Could you check a few things on this model? Use its own coordinates, in mm. Give positions to 0.01 mm unless a question says otherwise; leave off trailing zeros. Loops run counter-clockwise (first coordinate to the right, second up) from the corner with the lowest first, then second, coordinate; pieces in that order, holes last. Notation, with made-up numbers: (10.25, 30) - (52.25, 30) arc R11 ccw to (52.25, 34) - close; hole circle Ø7 at (-12, -1.5). An arc over 180 degrees is marked (long way). Write each question's results on one line, items separated by ' | '. Start each with the question number.
(1) Suppose I cut it at C-C (x = -19.5). Count the separate pieces of the cut face and the enclosed holes in it, and give its area (3 significant figures).
(2) Suppose I cut it at D-D (y = 1.5). Please give me the cut outline in (x, z) (1 decimal), and give its area (3 significant figures).
(3) Suppose I cut it at A-A (z = 8.5). Please give me the cut outline in (x, y), and give its area (3 significant figures).
(4) Suppose I cut it at B-B (y = 5.25). Please give me the cut outline in (x, z) (1 decimal).
(5) I need wall thicknesses on line 1 (Z direction, x = -19.5, y = 5); line 2 (X direction, y = 3.5, z = -13.5) (3 decimals); line 3 (X direction, y = 1.5, z = -14). Which ranges of each line are inside material? Lowest first, please.
(6) If we mould it in two halves opening along X, with no side actions, what happens to faces 1 (the face through (-6.331, 3.131, -14.795)), 2 (the face through (-13.7, 4.8, -13.9)), 3 (the face through (-16, 6.35, 0))? For each: released by +X, released by -X, zero draft, split by the parting line, or undercut.
(7) For pin 1 (7 mm diameter, centred on x = -20.18, z = -13.16, fed in from +Y); pin 2 (12.5 mm diameter, centred on x = -15.8, z = 5.57, fed in from -Y); pin 3 (12 mm diameter, centred on x = -13, z = -12, fed in from -Y), each with a flat end and sliding along its axis, tell me the tip position at first contact or that it passes through.
from build123d import *

# Parameters (mm, degrees)
BOSS_EXTRUDE1_DEPTH                               = 6.35
CSK_FOR_8_FLAT_HEAD_MACHINE_SCREW_100_D           = 4.4958
CSK_FOR_8_FLAT_HEAD_MACHINE_SCREW_100_CSINK_D     = 8.4328
CSK_FOR_8_FLAT_HEAD_MACHINE_SCREW_100_CSINK_ANGLE = 100
SKETCH2_R                                         = 82.042
CUT_EXTRUDE1_DEPTH                                = 43.217023873
SKETCH5_R                                         = 1.1303
CUT_EXTRUDE2_DEPTH                                = 35.271884391
SKETCH6_R                                         = 4.7625
CUT_EXTRUDE3_DEPTH                                = 35.271884391


with BuildPart() as part:
    # Sketch1 → Boss-Extrude1 (new body)
    with BuildSketch(Plane(origin=(0, 0, 0), x_dir=(1, 0, 0), z_dir=(0, 1, 0))):
        Polygon((-28.511825699, 11.575271113), (-22.161825699, 17.925271113), (-9.461825699, 17.925271113), (-3.111825699, 11.575271113), (-3.111825699, -12.554728887), (-28.511825699, -12.554728887), align=None)
    extrude(amount=BOSS_EXTRUDE1_DEPTH)

    # CSK for #8 Flat Head Machine Screw (100)1 (through all)
    with Locations(Plane(origin=(0, 6.35, 0), x_dir=(1, 0, 0), z_dir=(0, 1, 0))):
        with Locations((-20.177450699, 13.162771113), (-11.446200699, 13.162771113)):
            CounterSinkHole(CSK_FOR_8_FLAT_HEAD_MACHINE_SCREW_100_D / 2, CSK_FOR_8_FLAT_HEAD_MACHINE_SCREW_100_CSINK_D / 2, counter_sink_angle=CSK_FOR_8_FLAT_HEAD_MACHINE_SCREW_100_CSINK_ANGLE)

    # Sketch2 → Cut-Extrude1 (cut, through all)
    with BuildSketch(Plane.XY.offset(12.554728887)):
        with Locations((-15.811825699, -81.053067579)):
            Circle(SKETCH2_R)
    extrude(amount=-CUT_EXTRUDE1_DEPTH, mode=Mode.SUBTRACT)

    # Sketch5 → Cut-Extrude2 (cut, through all)
    with BuildSketch(Plane(origin=(0, 6.35, 0), x_dir=(1, 0, 0), z_dir=(0, 1, 0))):
        with Locations(Location((-15.799380503, -5.569728887, 0), (0, 0, 270))):
            Circle(SKETCH5_R)
    extrude(amount=-CUT_EXTRUDE2_DEPTH, mode=Mode.SUBTRACT)

    # Sketch6 → Cut-Extrude3 (cut, through all)
    with BuildSketch(Plane(origin=(0, 6.35, 0), x_dir=(1, 0, 0), z_dir=(0, 1, 0))):
        with Locations(Location((-15.799380503, -5.569728887, 0), (0, 0, 270))):
            Circle(SKETCH6_R)
    extrude(amount=-CUT_EXTRUDE3_DEPTH, mode=Mode.SUBTRACT)


solid = part.part
Output values:
1) separate pieces: 3 | enclosed holes: 0 | area: 107 mm2
2) outline: (-28.5, -11.6) - (-22.2, -17.9) - (-9.5, -17.9) - (-3.1, -11.6) - (-3.1, 12.6) - (-28.5, 12.6) - close; hole circle Ø4.5 at (-20.2, -13.2); hole circle Ø9.5 at (-15.8, 5.6); hole circle Ø4.5 at (-11.4, -13.2) | area: 631 mm2
3) outline: (-28.51, 0) arc R82.04 cw to (-19.55, 0.9) - (-19.55, 6.35) - (-28.51, 6.35) - close; (-12.05, 0.9) arc R82.04 cw to (-3.11, 0) - (-3.11, 6.35) - (-12.05, 6.35) - close | area: 104 mm2
4) outline: (-28.5, -11.6) - (-22.2, -17.9) - (-9.5, -17.9) - (-3.1, -11.6) - (-3.1, 12.6) - (-28.5, 12.6) - close; hole circle Ø5.8 at (-20.2, -13.2); hole circle Ø9.5 at (-15.8, 5.6); hole circle Ø5.8 at (-11.4, -13.2)
5) line 1: -17.93 to -15.68, -10.64 to 2.57, 8.57 to 12.55 | line 2: -26.587 to -22.4, -17.955 to -13.669, -9.224 to -5.037 | line 3: -26.09 to -22.26, -18.09 to -13.53, -9.36 to -5.54
6) face 1: released by +X | face 2: undercut | face 3: zero draft
7) pin 1: y = 5.75 | pin 2: y = 0.75 | pin 3: y = 0.51
